Geometry: see drawing. Coordinates: mm, zero at the bounding-box minimum. Round coordinates to 2 decimals unless told otherwise and drop trailing zeros. Order: outer loops, then holes, each group sorted by start corner. A loop starts at its lowest first (then second) coordinate and runs counter-clockwise, first axis right, second up.
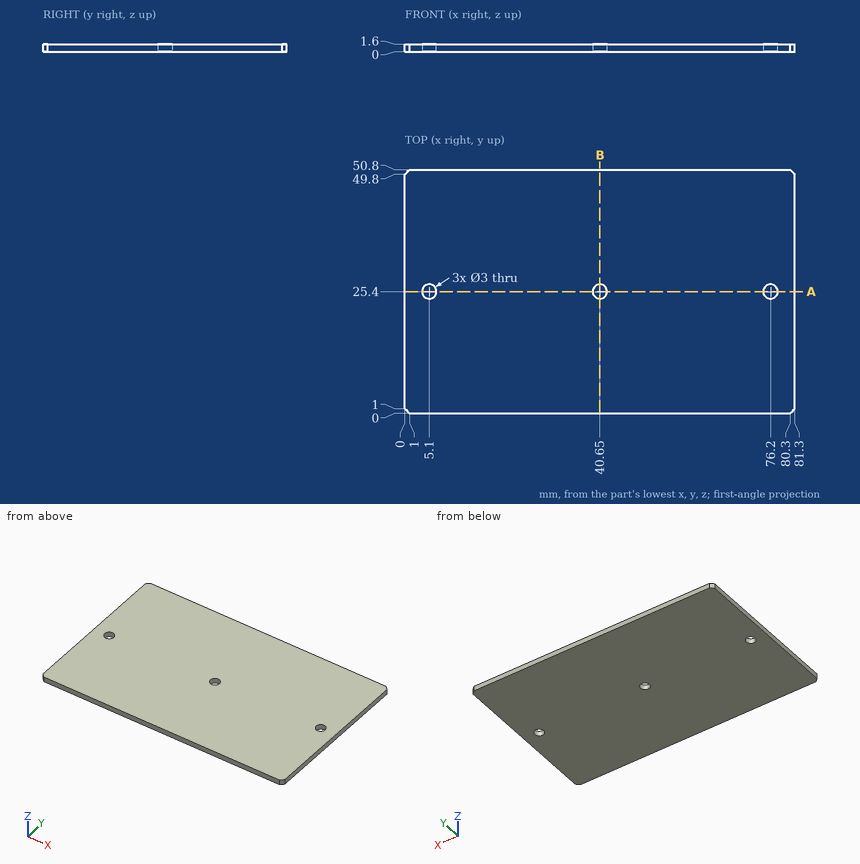
1. Section A-A on y = 25.4. Return loops of the section in (x, z), plus the area to 3 significant figures.
2. Line query: line 1 along Y through (x, z) = (40.65, 0.4); line 2 along Y through (x, z) = (6, 1.35). Output: solid intervals per line, ascending.
3. Section B-B on x = 40.65. Return loops of the section in (y, z).
Result:
1. outline: (0, 0) - (3.6, 0) - (3.6, 1.6) - (0, 1.6) - close; (6.6, 0) - (39.15, 0) - (39.15, 1.6) - (6.6, 1.6) - close; (42.15, 0) - (74.7, 0) - (74.7, 1.6) - (42.15, 1.6) - close; (77.7, 0) - (81.3, 0) - (81.3, 1.6) - (77.7, 1.6) - close
1. area: 116 mm2
2. line 1: y = 0 to 23.9, 26.9 to 50.8
2. line 2: y = 0 to 24.2, 26.6 to 50.8
3. outline: (0, 0) - (23.9, 0) - (23.9, 1.6) - (0, 1.6) - close; (26.9, 0) - (50.8, 0) - (50.8, 1.6) - (26.9, 1.6) - close
